```python
from build123d import *

# Parameters (mm, degrees)
SKETCH_1_W          = 80
SKETCH_1_H          = 60
EXTRUDE_1_DEPTH     = 10
SKETCH_2_R          = 5.5
CUT_EXTRUDE_1_DEPTH = 3.5
SKETCH_3_R          = 3
CUT_EXTRUDE_2_DEPTH = 51.990195136


with BuildPart() as part:
    # 草图1 → 凸台-拉伸1 (new body)
    with BuildSketch(Plane.XY):
        Rectangle(SKETCH_1_W, SKETCH_1_H)
    extrude(amount=EXTRUDE_1_DEPTH)

    # 草图2 → 切除-拉伸1 (cut)
    with BuildSketch(Plane.XY.offset(10)):
        with Locations((26, 16)):
            Circle(SKETCH_2_R)
        with Locations((26, -16)):
            Circle(SKETCH_2_R)
        with Locations((-26, 16)):
            Circle(SKETCH_2_R)
        with Locations((-26, -16)):
            Circle(SKETCH_2_R)
    extrude(amount=-CUT_EXTRUDE_1_DEPTH, mode=Mode.SUBTRACT)

    # 草图3 → 切除-拉伸2 (cut, through all)
    with BuildSketch(Plane.XY.offset(10)):
        with Locations((26, 16)):
            Circle(SKETCH_3_R)
        with Locations((26, -16)):
            Circle(SKETCH_3_R)
        with Locations((-26, 16)):
            Circle(SKETCH_3_R)
        with Locations((-26, -16)):
            Circle(SKETCH_3_R)
    extrude(amount=-CUT_EXTRUDE_2_DEPTH, mode=Mode.SUBTRACT)


solid = part.part
```
Read the model definition and answer for the solid it produces. Units are mm, in the model's axes. A direction names the side the tool comes from. Coordinates: 2 decimals unless noted, no trailing zeros. Loops run counter-clockwise (first coordinate to the right, second up) from the corner with the lowest first, then second, coordinate; pieces in that order, holes last. Notation, with made-up numbers: (32.5, 42) -> (38.5, 42) arc R7 ccw to (38.5, 52) -> close; hole circle Ø11 at (89, 41.25). An arc over 180 degrees is marked (long way). Return JSON: item names as keys, results as strings.
Item 1: Flat-ended cylindrical pins translate along their axes: P1, Ø5.5, axis at x = 25, y = 18.5, coming from the +Z side; P2, Ø9.5, axis at x = 26, y = 16, coming from the -Z side. Find the tip coordinate at first contact, or state that the pin passes through.
Answers:
{"P1": "stops at z = 6.5", "P2": "stops at z = 0"}
Item 2: Find section C-C (y = 16). Determine the outline of the cut face in (x, z), plus the area to 3 significant figures.
Answers:
{"outline": "(-40, 0) -> (-29, 0) -> (-29, 6.5) -> (-31.5, 6.5) -> (-31.5, 10) -> (-40, 10) -> close; (-23, 0) -> (23, 0) -> (23, 6.5) -> (20.5, 6.5) -> (20.5, 10) -> (-20.5, 10) -> (-20.5, 6.5) -> (-23, 6.5) -> close; (29, 0) -> (40, 0) -> (40, 10) -> (31.5, 10) -> (31.5, 6.5) -> (29, 6.5) -> close", "area": "645 mm2"}
Item 3: Find section A-A (x = -26). Determine the outline of the cut face in (y, z), plus the area to 3 significant figures.
Answers:
{"outline": "(-30, 0) -> (-19, 0) -> (-19, 6.5) -> (-21.5, 6.5) -> (-21.5, 10) -> (-30, 10) -> close; (-13, 0) -> (13, 0) -> (13, 6.5) -> (10.5, 6.5) -> (10.5, 10) -> (-10.5, 10) -> (-10.5, 6.5) -> (-13, 6.5) -> close; (19, 0) -> (30, 0) -> (30, 10) -> (21.5, 10) -> (21.5, 6.5) -> (19, 6.5) -> close", "area": "445 mm2"}
Item 4: For a pull along Y with two mould halves and no side action, classify faces 1 (the flat face through (-1, -30, 5)), 2 (the flat face through (-1, 0, 10)), 3 (the cylindrical face through (-27.19, 10.63, 8.27)) as +Y half, -Y half, draft (parallel to the pull), parting line (faces both ways), or undercut.
Answers:
{"face 1": "-Y half", "face 2": "draft", "face 3": "undercut"}
Item 5: Find section B-B (z = 1.25). Determine the outline of the cut face in (x, y), plus the area to 3 significant figures.
Answers:
{"outline": "(-40, -30) -> (40, -30) -> (40, 30) -> (-40, 30) -> close; hole circle Ø6 at (-26, -16); hole circle Ø6 at (-26, 16); hole circle Ø6 at (26, -16); hole circle Ø6 at (26, 16)", "area": "4,690 mm2"}
Item 6: For faces 4 (the cylindrical face through (-27.19, -21.37, 8.27)), 5 (the cylindrical face through (-26.65, -18.93, 3.3)), determine the directions among +Z, -Z, +X, -X, +Y, -Y from which every point of the face is accessible in a straight line to the end or side of a thin tool.
Answers:
{"face 4": "+Z", "face 5": "+Z, -Z"}
Item 7: Find the intervals of material crossed by probe 1 along Y at (x, z) = (-26, 8.75); probe 2 along Y at (x, z) = (26, 2); probe 3 along X at (y, z) = (-18.5, 1.25), in increasing order.
Answers:
{"probe 1": "y = -30 to -21.5, -10.5 to 10.5, 21.5 to 30", "probe 2": "y = -30 to -19, -13 to 13, 19 to 30", "probe 3": "x = -40 to -27.66, -24.34 to 24.34, 27.66 to 40"}
